For this review, take the finished solid that the model builds, in its own axes (mm). A direction names the side the tool comes from. Give positions to 0.01 mm unless a question says otherwise; leave off trailing zeros. Order: outer loops, then holes, each group sorted by start corner. A loop starts at its lowest first (then second) coordinate and runs counter-clockwise, first axis right, second up. Notation, with made-up numbers: (-22, 68) -> (28, 68) arc R24 cw to (28, 105) -> close; hole circle Ø9 at (48.25, 1). An arc over 180 degrees is marked (long way). Return JSON: item names as keys, results as strings. Group by question number.
1) Insertion check: P1, Ø22, axis at x = 54.5, z = 40.5, coming from the +Y side; P2, Ø1, axis at x = -8, z = 49, coming from the +Y side (3 decimals); P3, Ø19, axis at y = -15, z = 14, coming from the -X side (3 decimals); P4, Ø3, axis at y = 18.5, z = 30, coming from the -X side. Each pin has a flat end and moves straight along its axis. Give the tip position at first contact, or say it passes through.
2) Add section B-B (y = 48.5). Give the boundary of the cut face in (x, z) (3 decimals), then the cut area to 3 significant figures.
3) To check wall thickness, follow line 1 along X through (y, z) = (53.5, 9) (3 decimals); line 2 along Y through (x, z) = (-22, 17) (3 decimals); line 3 along Z through (x, y) = (-2.5, 7) (3 decimals). State the ranges of each line that lie inside material, in increasing order.
4) For faces 1 (the face through (46, 25.4, 42)), 2 (the face through (32.57, -14.44, 51.81)), 3 (the face through (-4, 3.175, 36)), list the 3-axis set-ups (+Z, -Z, +X, -X, +Y, -Y) from which the entire face can be reached by the end or side of a thin tool; tool diameter is ignored.
5) Add section A-A (x = 81). Give the boundary of the cut face in (y, z) (3 decimals), then the cut area to 3 significant figures.
from build123d import *

# Parameters (mm, degrees)
F1_DEPTH    = 63.5
F0_W        = 25.4
F0_H        = 19.05
F0_H_2      = 4.7498
F0_H_3      = 4.7752
F2_DEPTH    = 25.4
F4_DEPTH    = 3.175
F5_T1_DEPTH = 100.3187641102
F5_T3_DEPTH = 57.15
F5_T6_ANGLE = 180


# Not quite as in the source:
# - a fillet or chamfer that OpenCascade refuses, or shapes differently, is made with other operations: its cross-section is extruded or revolved along the edge and cut away or added


with BuildPart() as f1:
    # F0 (on Front) → F1 (new body, symmetric)
    with BuildSketch(Plane.XZ):
        Polygon((41.275, -9.525), (41.275, 9.525), (22.225, 9.525), (-41.275, 9.525), (-41.275, -9.525), align=None)
    extrude(amount=F1_DEPTH, both=True)

    # F0 (on Front) → F2 (join, symmetric)
    with BuildSketch(Plane.XZ):
        with BuildLine():
            Line((22.225, 9.525), (41.275, 9.525))
            Line((41.275, 9.525), (41.275, 27.0002))
            ThreePointArc((41.275, 27.0002), (45.9246798487, 38.2255201513), (57.15, 42.8752))
            Line((57.15, 42.8752), (60.325, 42.8752))
            Line((60.325, 42.8752), (60.325, 61.9252))
            Line((60.325, 61.9252), (57.15, 61.9252))
            add(Edge.make_bspline(
                [(56.7157172379, 61.9224998023), (56.8604203243, 61.9234406697), (57.0051814864, 61.9243403706), (57.15, 61.9252)],
                knots=[111.1645323541, 111.1645323541, 111.1645323541, 111.1645323541, 111.5045361635, 111.5045361635, 111.5045361635, 111.5045361635], degree=3))
            ThreePointArc((56.7157172379, 61.9224998023), (32.3012278929, 51.5418818855), (22.225, 27.0002))
            Line((22.225, 27.0002), (22.225, 9.525))
        make_face()
        with Locations((73.025, 52.4002)):
            Rectangle(F0_W, F0_H)
        with Locations((73.025, 64.3001)):
            Rectangle(F0_W, F0_H_2)
        with Locations((73.025, 40.4876)):
            Rectangle(F0_W, F0_H_3)
    extrude(amount=F2_DEPTH, both=True)

    # F0 (on Front) → F3 (revolve)
    with BuildSketch(Plane.XZ):
        Polygon((85.725, 61.9252), (85.725, 42.8752), (85.725, 38.1), (111.125, 38.1), (111.125, 66.675), (85.725, 66.675), align=None)
    revolve(axis=Axis((85.725, 0, 52.3875), (0, 0, 1)))

    # F0 (on Front) → F4 (join, symmetric)
    with BuildSketch(Plane.XZ):
        with BuildLine():
            Line((-41.275, 9.525), (22.225, 9.525))
            Line((22.225, 9.525), (22.225, 27.0002))
            ThreePointArc((22.225, 27.0002), (32.3012278929, 51.5418818855), (56.7157172379, 61.9224998023))
            add(Edge.make_bspline(
                [(-41.275, 9.525), (-31.6977544753, 56.9066902811), (9.4049210672, 61.6148824052), (56.7157172379, 61.9224998023)],
                knots=[0, 0, 0, 0, 111.1645323541, 111.1645323541, 111.1645323541, 111.1645323541], degree=3))
        make_face()
    extrude(amount=F4_DEPTH, both=True)

    # F5: fillet of radius 12.7 on 4 edges, made by hand

    # F5_s2 → F5_t1 (cut)
    with BuildSketch(Plane.XZ.offset(-50.1593820551)):
        with BuildLine():
            ThreePointArc((70.228752822, 66.675), (64.7368287512, 65.4261471041), (60.325, 61.9252))
            Line((60.325, 61.9252), (60.325, 66.675))
            Line((60.325, 66.675), (70.228752822, 66.675))
        make_face()
    extrude(amount=F5_T1_DEPTH, mode=Mode.SUBTRACT)

    # F5_s4 → F5_t3 (cut)
    with BuildSketch(Plane.YZ.offset(28.575)):
        with BuildLine():
            ThreePointArc((-25.4, 53.975), (-21.6802561211, 62.9552561211), (-12.7, 66.675))
            Line((-12.7, 66.675), (-25.4, 66.675))
            Line((-25.4, 66.675), (-25.4, 53.975))
        make_face()
        with BuildLine():
            ThreePointArc((25.4, 53.975), (21.6802561211, 62.9552561211), (12.7, 66.675))
            Line((12.7, 66.675), (25.4, 66.675))
            Line((25.4, 66.675), (25.4, 53.975))
        make_face()
    extrude(amount=F5_T3_DEPTH, mode=Mode.SUBTRACT)

    # F5_s5 → F5_t6 (revolve, cut)
    with BuildSketch(Plane.YZ.offset(85.725)):
        with BuildLine():
            ThreePointArc((25.4, 53.975), (21.6802561211, 62.9552561211), (12.7, 66.675))
            Line((12.7, 66.675), (25.4, 66.675))
            Line((25.4, 66.675), (25.4, 53.975))
        make_face()
    revolve(axis=Axis((85.725, 0, 66.675), (0, 0, -1)), revolution_arc=F5_T6_ANGLE, mode=Mode.SUBTRACT)


solid = f1.part
Evaluation:
{
 "1": {"P1": "y = 25.4", "P2": "y = 3.175", "P3": "x = -41.275", "P4": "x = 22.26"},
 "2": {"outline": "(-41.275, -9.525) -> (41.275, -9.525) -> (41.275, 9.525) -> (-41.275, 9.525) -> close", "area": "1,570 mm^2"},
 "3": {"line 1": "-41.275 to 41.275", "line 2": "-3.175 to 3.175", "line 3": "-9.525 to 9.525"},
 "4": {"face 1": "+Z, +X, -X, +Y", "face 2": "+Z, -X, -Y", "face 3": "+Z, -X, +Y"},
 "5": {"outline": "(-25.4, 38.1) -> (25.4, 38.1) -> (25.4, 53.975) arc R12.7 ccw to (12.7, 66.675) -> (-12.7, 66.675) arc R12.7 ccw to (-25.4, 53.975) -> close", "area": "1,380 mm^2"}
}
